The figure shows three views and two pictorial views of one solid part (mm, origin at its lowest corner). Answer the questions. A direction names the side the tool comes from. Round coordinates to 2 decimals unless told otherwise and drop trailing zeros. Write each loop counter-clockwise with the first axis right and the second up, starting at its lowest first coordinate (ties: lowest second). Pieces come first, ordered by that corner, then holes.
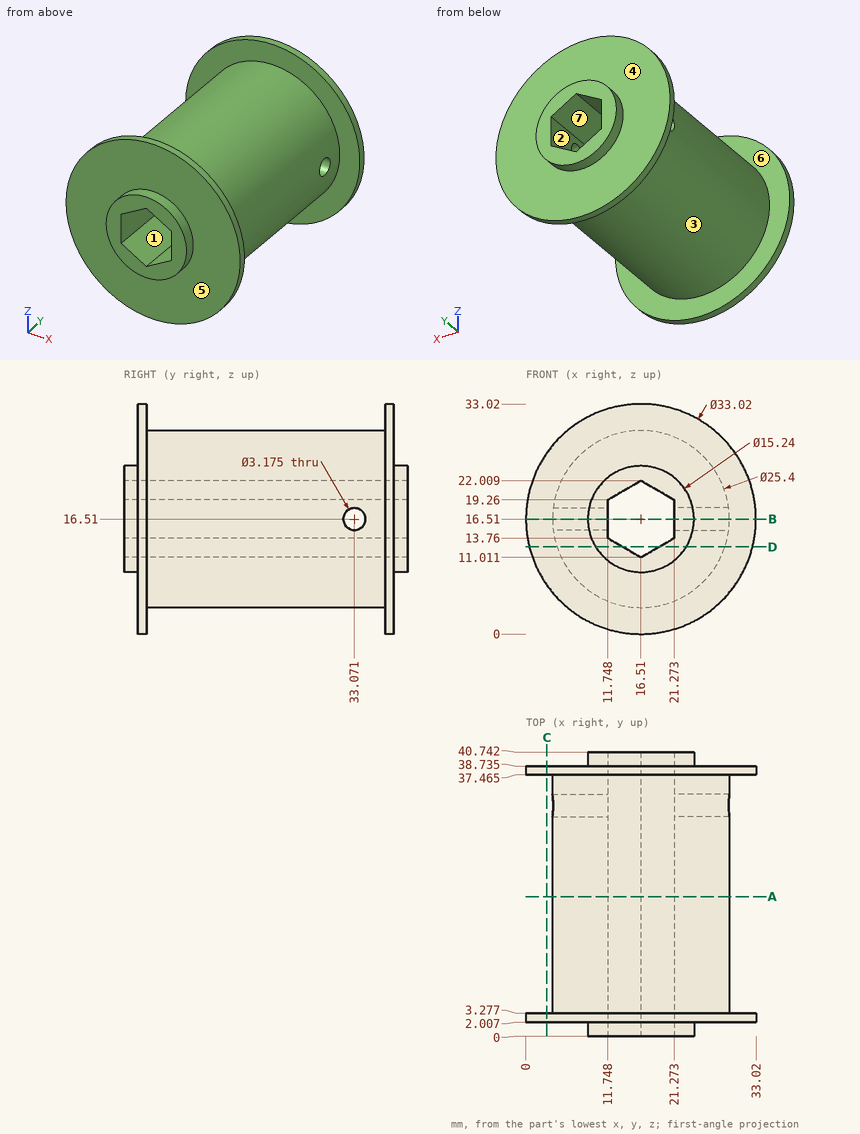
Q1. Determine the mould class of the marked faces 1, 2, 3 and 4 for opening direction Z: pulls with the +Z half, pulls with the -Z half, needs draft (parallel to the pull), parting line crosses it, or undercut.
Verdict:
face 1: undercut
face 2: undercut
face 3: parting line crosses it
face 4: needs draft
Q2. Section B-B (z = 16.51) is taken. State how many separate pieces and enclosed holes the cut face has, then the cut area to 3 significant figures.
Verdict:
separate pieces: 4
enclosed holes: 0
area: 575 mm2
Q3. Section C-C (x = 3) is taken. Determine the outline of the cut face in (y, z) (1 decimal).
Verdict:
outline: (2, 7) - (3.3, 7) - (3.3, 26) - (2, 26) - close; (37.5, 7) - (38.7, 7) - (38.7, 26) - (37.5, 26) - close
Q4. Section D-D (z = 12.5) is taken. Determine the outline of the cut face in (x, y) (1 decimal), then the cut area to 3 significant figures.
Verdict:
outline: (0.5, 2) - (10, 2) - (10, 0) - (13.9, 0) - (13.9, 40.7) - (10, 40.7) - (10, 38.7) - (0.5, 38.7) - (0.5, 37.5) - (4.5, 37.5) - (4.5, 3.3) - (0.5, 3.3) - close; (19.1, 0) - (23, 0) - (23, 2) - (32.5, 2) - (32.5, 3.3) - (28.6, 3.3) - (28.6, 37.5) - (32.5, 37.5) - (32.5, 38.7) - (23, 38.7) - (23, 40.7) - (19.1, 40.7) - close
area: 747 mm2
Q5. Straight lines are drawn through the part: probe 1 along Y at (x, z) = (26.5, 16.51) (1 decimal); probe 2 along Y at (x, z) = (27, 27) (1 decimal); probe 3 along Y at (x, z) = (8.5, 26) (1 decimal). For each, find the intervals that lie inside material, in ascending order.
Verdict:
probe 1: y = 2 to 31.5, 34.7 to 38.7
probe 2: y = 2 to 3.3, 37.5 to 38.7
probe 3: y = 2 to 38.7
Q6. Flat-ended cylindrical pins translate along their axes: pin 1 Ø1.6 at (y, z) = (12, 16) entering from -X; pin 2 Ø4 at (y, z) = (33.07, 16.51) entering from +X; pin 3 Ø8 at (x, y) = (10.5, 18.5) entering from +Z. Find the tip coordinate at first contact, or state that the pin passes through.
Verdict:
pin 1: stops at x = 3.81
pin 2: stops at x = 29.21
pin 3: stops at z = 29.05
Q7. Section A-A (y = 20) is taken. Determine the outline of the cut face in (x, z), then the cut area to 3 significant figures.
Verdict:
outline: circle Ø25.4 at (16.51, 16.51); hole (11.75, 13.76) - (16.51, 11.01) - (21.27, 13.76) - (21.27, 19.26) - (16.51, 22.01) - (11.75, 19.26) - close
area: 428 mm2
Q8. Which of the six approach directions +Z, -Z, +X, -X, +Y, -Y give full straight-line access (tool end or side, diameter ignored) to the marked faces 5, 6 and 7?
Verdict:
face 5: -Y
face 6: none
face 7: +Y, -Y
